Could you check a few things on this model? Use its own coordinates, in mm. A direction names the side the tool comes from. Give positions to 0.01 mm unless a question says otherwise; leave off trailing zeros. Order: outer loops, then holes, each group sorted by start corner. A loop starts at its lowest first (then second) coordinate and runs counter-clockwise, first axis right, second up.
(1) If I drill on probe 1 along X at (y, z) = (-99, 3.9); probe 2 along Y at (x, z) = (-150, 3.9); probe 3 along X at (y, z) = (-133, 7.5), over which ranges is the centre line in solid material (lowest first)?
(2) Will these pins go through, and if not, where does the flat tip stop? pin 1 (5 mm diameter, centred on x = -150, y = -183, fed in from +Z); pin 2 (4 mm diameter, centred on y = -171, z = 2, fed in from +X); pin 3 (2.5 mm diameter, centred on x = 19.5, y = -99, fed in from +Z).
(3) On a 3-axis mill with a long thin cutter (end or side, diameter ignored), from which of +Z, -Z, +X, -X, +Y, -Y can I reach the whole of each face in a straight line? I mean faces 1 (the flat face through (201, -90, 4)), 2 (the flat face through (110.5, -128, 4)). Say none if no direction works.
(4) Imagine slicing it at B-B, the plane y = -165. Write out the boundary of the cut face in (x, z), then the cut area to 3 significant figures.
(5) If we mould it in two halves opening along X, with no side actions, what happens to faces 3 (the flat face through (-162, -122, 4)), 4 (the flat face through (17, -49, 4)), 5 (the cylindrical face through (107.34, -147.51, 4.06))? For each: released by +X, released by -X, zero draft, split by the parting line, or undercut.
(6) Imagine slicing it at A-A, the plane z = 2.25. State how many separate pieces and enclosed holes the cut face has, then the cut area to 3 significant figures.
from build123d import *

# Parameters (mm, degrees)
BOSS_EXTRU_1_DEPTH                                 = 8
ESQUISSE2_R                                        = 15
ESQUISSE2_R_2                                      = 1.5
ENL_V_MAT_EXTRU_1_DEPTH                            = 9
CHAMBRAGE_POUR_VIS_T_TE_CYLINDRIQUE_CO_D           = 3
CHAMBRAGE_POUR_VIS_T_TE_CYLINDRIQUE_CO_CBORE_D     = 5.5
CHAMBRAGE_POUR_VIS_T_TE_CYLINDRIQUE_CO_CBORE_DEPTH = 2


with BuildPart() as part:
    # Esquisse1 → Boss.-Extru.1 (new body)
    with BuildSketch(Plane.XY):
        with BuildLine():
            Line((-162, -49), (201, -49))
            Line((201, -49), (201, -133))
            ThreePointArc((201, -133), (183.426406871, -175.426406871), (141, -193))
            Line((141, -193), (-162, -193))
            Line((-162, -193), (-162, -49))
        make_face()
    extrude(amount=BOSS_EXTRU_1_DEPTH)

    # Esquisse2 → Enlèv. mat.-Extru.1 (cut, through all)
    with BuildSketch(Plane.XY.offset(8)):
        with Locations((-52, -128)):
            Circle(ESQUISSE2_R)
        with Locations((122.5, -128)):
            Circle(ESQUISSE2_R_2)
        with BuildLine():
            Line((76, -150.5), (100, -150.5))
            ThreePointArc((100, -150.5), (107.424621202, -147.424621202), (110.5, -140))
            Line((110.5, -140), (110.5, -116))
            ThreePointArc((110.5, -116), (107.424621202, -108.575378798), (100, -105.5))
            Line((100, -105.5), (76, -105.5))
            ThreePointArc((76, -105.5), (68.575378798, -108.575378798), (65.5, -116))
            Line((65.5, -116), (65.5, -140))
            ThreePointArc((65.5, -140), (68.575378798, -147.424621202), (76, -150.5))
        make_face()
    extrude(amount=-ENL_V_MAT_EXTRU_1_DEPTH, mode=Mode.SUBTRACT)

    # Chambrage pour vis à tête cylindrique courte six pans creux M31 (through all)
    with Locations(Plane.XY.offset(8)):
        with Locations((-150, -99), (19.5, -99), (189, -99), (-150, -183), (19.5, -183), (127, -183)):
            CounterBoreHole(CHAMBRAGE_POUR_VIS_T_TE_CYLINDRIQUE_CO_D / 2, CHAMBRAGE_POUR_VIS_T_TE_CYLINDRIQUE_CO_CBORE_D / 2, CHAMBRAGE_POUR_VIS_T_TE_CYLINDRIQUE_CO_CBORE_DEPTH)


solid = part.part
Answer block:
1. probe 1: x = -162 to -151.5, -148.5 to 18, 21 to 187.5, 190.5 to 201
1. probe 2: y = -193 to -184.5, -181.5 to -100.5, -97.5 to -49
1. probe 3: x = -162 to -66.14, -37.86 to 65.5, 110.5 to 201
2. pin 1: stops at z = 6
2. pin 2: stops at x = 189
2. pin 3: passes through
3. face 1: +Z, -Z, +X, +Y, -Y
3. face 2: +Z, -Z
4. outline: (-162, 0) - (191.75, 0) - (191.75, 8) - (-162, 8) - close
4. area: 2,830 mm2
5. face 3: released by -X
5. face 4: zero draft
5. face 5: undercut
6. separate pieces: 1
6. enclosed holes: 9
6. area: 48,800 mm2
